```python
from build123d import *

# Parameters (mm, degrees)
BOSS_EXTRU_3_DEPTH = 2.2
BOSS_EXTRU_3_DRAFT = 10
BOSS_EXTRU_4_DEPTH = 3.6


with BuildPart() as part:
    # Esquisse2 → Boss.-Extru.3 (with draft: the straight prism first)
    with BuildSketch(Plane.XY):
        with BuildLine():
            ThreePointArc((59.333408072, 1.170179372), (59.626301291, 0.463072591), (60.333408072, 0.170179372))
            Line((60.333408072, 0.170179372), (61.407735426, 0.170179372))
            ThreePointArc((61.407735426, 0.170179372), (62.114842207, 0.463072591), (62.407735426, 1.170179372))
            Line((62.407735426, 1.170179372), (62.407735426, 4.679932735))
            Line((62.407735426, 4.679932735), (63.46838565, 4.679932735))
            ThreePointArc((63.46838565, 4.679932735), (64.175492431, 4.972825954), (64.46838565, 5.679932735))
            Line((64.46838565, 5.679932735), (64.46838565, 6.043946188))
            ThreePointArc((64.46838565, 6.043946188), (64.175492431, 6.75105297), (63.46838565, 7.043946188))
            Line((63.46838565, 7.043946188), (62.407735426, 7.043946188))
            Line((62.407735426, 7.043946188), (62.407735426, 18.788901345))
            ThreePointArc((62.407735426, 18.788901345), (62.114842207, 19.496008126), (61.407735426, 19.788901345))
            Line((61.407735426, 19.788901345), (60.146458975, 19.788901345))
            ThreePointArc((60.146458975, 19.788901345), (59.625963925, 19.642766032), (59.257594289, 19.24707115))
            Line((59.257594289, 19.24707115), (52.985126346, 7.078274373))
            ThreePointArc((52.985126346, 7.078274373), (52.902171942, 6.855832499), (52.873991031, 6.620104568))
            Line((52.873991031, 6.620104568), (52.873991031, 5.679932735))
            ThreePointArc((52.873991031, 5.679932735), (53.16688425, 4.972825954), (53.873991031, 4.679932735))
            Line((53.873991031, 4.679932735), (59.333408072, 4.679932735))
            Line((59.333408072, 4.679932735), (59.333408072, 2.689573991))
            Line((59.333408072, 2.689573991), (59.333408072, 1.170179372))
        make_face()
        Polygon((59.823459842, 7.043946188), (59.823459842, 14.963775897), (55.741143498, 7.043946188), align=None, mode=Mode.SUBTRACT)
    extrude(amount=BOSS_EXTRU_3_DEPTH)
    # Boss.-Extru.3: the draft: its side faces are tilted about the plane it starts from
    boss_extru_3_sides = [part.faces().sort_by_distance(p)[0] for p in [
        (60.777097201, 19.788901345, 1.1),
        (59.823459842, 11.003861043, 1.1),
        (57.78230167, 11.003861043, 1.1),
        (57.78230167, 7.043946188, 1.1),
        (62.407735426, 12.916423767, 1.1),
        (62.938060538, 7.043946188, 1.1),
        (64.175492431, 6.75105297, 1.1),
        (64.46838565, 5.861939462, 1.1),
        (64.175492431, 4.972825954, 1.1),
        (62.938060538, 4.679932735, 1.1),
        (62.407735426, 2.925056054, 1.1),
        (62.114842207, 0.463072591, 1.1),
        (60.870571749, 0.170179372, 1.1),
        (59.626301291, 0.463072591, 1.1),
        (59.333408072, 2.925056054, 1.1),
        (56.603699552, 4.679932735, 1.1),
        (53.16688425, 4.972825954, 1.1),
        (52.873991031, 6.150018652, 1.1),
        (52.902171942, 6.855832499, 1.1),
        (56.121360317, 13.162672762, 1.1),
        (59.625963925, 19.642766032, 1.1),
        (62.114842207, 19.496008126, 1.1),
    ]]
    draft(boss_extru_3_sides, Plane.XY, BOSS_EXTRU_3_DRAFT)

    # Esquisse3 → Boss.-Extru.4 (add)
    with BuildSketch(Plane.XY):
        with BuildLine():
            Line((60.157735426, 19.329540359), (61.457735426, 19.329540359))
            ThreePointArc((61.457735426, 19.329540359), (62.257735426, 18.529540359), (61.457735426, 17.729540359))
            Line((61.457735426, 17.729540359), (60.157735426, 17.729540359))
            ThreePointArc((60.157735426, 17.729540359), (59.357735426, 18.529540359), (60.157735426, 19.329540359))
        make_face()
        with BuildLine():
            Line((60.157735426, 2.229540359), (61.457735426, 2.229540359))
            ThreePointArc((61.457735426, 2.229540359), (62.257735426, 1.429540359), (61.457735426, 0.629540359))
            Line((61.457735426, 0.629540359), (60.157735426, 0.629540359))
            ThreePointArc((60.157735426, 0.629540359), (59.357735426, 1.429540359), (60.157735426, 2.229540359))
        make_face()
    extrude(amount=-BOSS_EXTRU_4_DEPTH)


solid = part.part
```
Source: CAD feature listing. Evaluate the final solid. Frame: model axes, mm. A direction names the side the tool comes from. Give positions to 0.01 mm unless a question says otherwise; leave off trailing zeros. Loops run counter-clockwise (first coordinate to the right, second up) from the corner with the lowest first, then second, coordinate; pieces in that order, holes last. Notation, with made-up numbers: (52.25, 18) -> (75.25, 18) arc R26 cw to (75.25, 50) -> close; hole circle Ø7 at (45, -1). An arc over 180 degrees is marked (long way). Put each result on its own line as item: value. Start each with the question number.
1) Cut plane D-D (y = 3.25). Return loops of the section in (x, z).
2) Contact query for flat-ended pins moving along their axis: P1, Ø1, axis at y = 10, z = 1.5, coming from the +X side; P2, Ø3, axis at y = 13.5, z = -0.5, coming from the +X side; P3, Ø1, axis at x = 61, z = -1, coming from the +Y side. Output: stop coordinate, or through.
3) Draft query along Y for faces 1 (the face through (57, 10, 0)), 2 (the face through (61.97, 0.59, 1.08)), 3 (the face through (64.047, 6.61, 1.085)). Return one class per face: released by +Y, released by -Y, zero draft, split by the parting line, or undercut.
4) Cut plane B-B (x = 58). Return loops of the section in (y, z), then the cut area to 3 significant figures.
5) Cut plane A-A (z = -1.2). Return loops of the section in (x, y), then the cut area to 3 significant figures.
6) Reachability of faces 4 (the face through (62.258, 1.447, -1.775)), 5 (the face through (56.76, 4.87, 1.08)), 6 (the face through (61, 2.23, -2)) from +Z, -Z, +X, -X, +Y, -Y: full face, straight path, thin tool, end or side. Return the list, or none.
7) Cut plane C-C (z = 1.8). Return loops of the section in (x, y).
8) Material intervals for probe 1 along Y at (x, z) = (60.5, -3.25); probe 2 along Y at (x, z) = (61.75, -1.45); probe 3 along X at (y, z) = (10.75, 0.2), sorted ascending.
Results are:
1. outline: (59.33, 0) -> (62.41, 0) -> (62.02, 2.2) -> (59.72, 2.2) -> close
2. P1: stops at x = 62.23
2. P2: stops at x = 62.41
2. P3: stops at y = 19.33
3. face 1: undercut
3. face 2: released by -Y
3. face 3: released by +Y
4. outline: (4.68, 0) -> (7.04, 0) -> (6.66, 2.2) -> (5.07, 2.2) -> close; (11.43, 0) -> (16.81, 0) -> (15.96, 2.2) -> (12.27, 2.2) -> close
4. area: 14.3 mm2
5. outline: (60.16, 0.63) -> (61.46, 0.63) arc R0.8 ccw to (61.46, 2.23) -> (60.16, 2.23) arc R0.8 ccw to start; (60.16, 17.73) -> (61.46, 17.73) arc R0.8 ccw to (61.46, 19.33) -> (60.16, 19.33) arc R0.8 ccw to start
5. area: 8.18 mm2
6. face 4: -Z, +X
6. face 5: +Z, -X, -Y
6. face 6: -Z, +X, -X
7. outline: (53.19, 5.68) arc R0.68 ccw to (53.87, 5) -> (59.65, 5) -> (59.65, 1.17) arc R0.68 ccw to (60.33, 0.49) -> (61.41, 0.49) arc R0.68 ccw to (62.09, 1.17) -> (62.09, 5) -> (63.47, 5) arc R0.68 ccw to (64.15, 5.68) -> (64.15, 6.04) arc R0.68 ccw to (63.47, 6.73) -> (62.09, 6.73) -> (62.09, 18.79) arc R0.68 ccw to (61.41, 19.47) -> (60.15, 19.47) arc R0.68 ccw to (59.54, 19.1) -> (53.27, 6.93) arc R0.68 ccw to (53.19, 6.62) -> close; hole (55.22, 6.73) -> (60.14, 6.73) -> (60.14, 16.27) -> close
8. probe 1: y = 0.63 to 2.23, 17.73 to 19.33
8. probe 2: y = 0.68 to 2.17, 17.78 to 19.27
8. probe 3: x = 54.92 to 57.61, 59.86 to 62.37
